from build123d import *

# Parameters (mm, degrees)
SKETCH4_W                                           = 12
SKETCH4_H                                           = 7.5
BOSS_EXTRUDE1_DEPTH                                 = 100
CUT_EXTRUDE1_DEPTH                                  = 101.460191121
FILLET1_R                                           = 0.2
CHAMFER1_SIZE                                       = 0.7
CHAMFER2_SIZE                                       = 0.8
CBORE_FOR_M3_HEX_SOCKET_HEAD_CAP_SCREW1_D           = 3.5
CBORE_FOR_M3_HEX_SOCKET_HEAD_CAP_SCREW1_CBORE_D     = 6
CBORE_FOR_M3_HEX_SOCKET_HEAD_CAP_SCREW1_CBORE_DEPTH = 4.4
LPATTERN1_COUNT                                     = 5
LPATTERN1_PITCH                                     = 20


with BuildPart() as part:
    # Sketch4 → Boss-Extrude1 (new body)
    with BuildSketch(Plane.XY):
        with Locations((0, -3.75)):
            Rectangle(SKETCH4_W, SKETCH4_H)
    extrude(amount=BOSS_EXTRUDE1_DEPTH)

    # Sketch5 → Cut-Extrude1 (cut, through all)
    with BuildSketch(Plane.XY):
        with BuildLine():
            ThreePointArc((-5.329252402, -1.887480513), (-7.9134, -2.3), (-5.329252402, -2.712519487))
            ThreePointArc((-5.329252402, -2.712519487), (-5.158134449, -2.549348252), (-4.927570698, -2.601755909))
            ThreePointArc((-4.927570698, -2.601755909), (-4.265, -2.3), (-4.927570698, -1.998244091))
            ThreePointArc((-4.927570698, -1.998244091), (-5.158134449, -2.050651748), (-5.329252402, -1.887480513))
        make_face()
    cut_extrude1 = extrude(amount=CUT_EXTRUDE1_DEPTH, mode=Mode.SUBTRACT)

    # Mirror3: Cut-Extrude1 across plane
    add(cut_extrude1.mirror(Plane(origin=(0, 0, 0), x_dir=(0, 0, 1), z_dir=(1, 0, 0))), mode=Mode.SUBTRACT)

    # Fillet1
    fillet1_edges = [part.edges().sort_by_distance(p)[0] for p in [
        (-6, -3.487185933, 50),
        (-6, -1.112814067, 50),
        (6, -1.112814067, 50),
        (6, -3.487185933, 50),
    ]]
    fillet(fillet1_edges, radius=FILLET1_R)

    # Chamfer1
    chamfer1_edges = [part.edges().sort_by_distance(p)[0] for p in [
        (-6, 0, 50),
        (6, 0, 50),
    ]]
    chamfer(chamfer1_edges, length=CHAMFER1_SIZE)

    # Chamfer2
    chamfer2_edges = [part.edges().sort_by_distance(p)[0] for p in [
        (6, -7.5, 50),
        (-6, -7.5, 50),
    ]]
    chamfer(chamfer2_edges, length=CHAMFER2_SIZE)

    # CBORE for M3 Hex Socket Head Cap Screw1 (through all)
    with Locations(Plane(origin=(0, 0, 0), x_dir=(1, 0, 0), z_dir=(0, 1, 0))):
        with Locations((0, -10)):
            cbore_for_m3_hex_socket_head_cap_screw1 = CounterBoreHole(CBORE_FOR_M3_HEX_SOCKET_HEAD_CAP_SCREW1_D / 2, CBORE_FOR_M3_HEX_SOCKET_HEAD_CAP_SCREW1_CBORE_D / 2, CBORE_FOR_M3_HEX_SOCKET_HEAD_CAP_SCREW1_CBORE_DEPTH)

    # LPattern1: CBORE for M3 Hex Socket Head Cap Screw1 ×5
    with Locations(*[(0, 0, i * LPATTERN1_PITCH) for i in range(1, LPATTERN1_COUNT)]):
        add(cbore_for_m3_hex_socket_head_cap_screw1, mode=Mode.SUBTRACT)


solid = part.part
Input: part model. Units: mm. Frame: model coordinates. A direction names the side the tool comes from. Give positions to 0.01 mm unless a question says otherwise; leave off trailing zeros. Use one line per item in the form item = value. Start each with the question number.
1) Ray query, probe 1 along X at (y, z) = (-1.05, 70); probe 2 along X at (y, z) = (-5.8, 70); probe 3 along X at (y, z) = (-2.3, 78) (3 decimals). Return the intervals inside material, ascending. Write a range as from..to.
2) Pin query (flat end, axial travel): pin 1 (1.8 mm diameter, centred on x = 0.5, z = 71.5, fed in from +Y). Return the tip coordinate at first contact, or that it passes through.
3) Set-up query: faces 4 (the cylindrical face through (0.228, -5.972, 8.265)), 5 (the flat face through (2, -4.4, 70)). Return all of +Z, -Z, +X, -X, +Y, -Y with unobstructed straight access to the full face (end or side cutting, diameter ignored); none if empty.
4) Section query A-A on x = 0. Count the separate pieces of the cut face and the enclosed holes in it, then the cut area to 3 significant figures.
5) Draft query along X for faces 1 (the flat face through (-4, 0, 49)), 2 (the cylindrical face through (0.38, -5.97, 91.71)), 3 (the flat face through (6, -5, 49)). Return one class per face: pulls with the +X half, pulls with the -X half, needs draft (parallel to the pull), parting line crosses it, or undercut.
Outcome:
q1.probe_1 = -5.99..-3, 3..5.99
q1.probe_2 = -6..-1.75, 1.75..6
q1.probe_3 = -4.265..4.265
q2.pin_1 = -4.4
q3.face_4 = +Y, -Y
q3.face_5 = +Y
q4.separate_pieces = 6
q4.enclosed_holes = 0
q4.area = 564 mm^2
q5.face_1 = needs draft
q5.face_2 = undercut
q5.face_3 = pulls with the +X half
